Geometry check sheet. Reference: the model listing, model coordinates, mm. A direction names the side the tool comes from. Give positions to 0.01 mm unless a question says otherwise; leave off trailing zeros. Loops run counter-clockwise (first coordinate to the right, second up) from the corner with the lowest first, then second, coordinate; pieces in that order, holes last. Notation, with made-up numbers: (17.5, -1) - (62.5, -1) arc R10 cw to (62.5, 10) - close; hole circle Ø9 at (-14, 57). An arc over 180 degrees is marked (long way). One line per question, with ' | ' between items. Start each with the question number.
from build123d import *

# Parameters (mm, degrees)
SKETCH1_R           = 7.5
SKETCH1_W           = 30
SKETCH1_H           = 3
SKETCH1_W_2         = 3
SKETCH1_H_2         = 30
BOSS_EXTRUDE2_DEPTH = 70


with BuildPart() as part:
    # Sketch1 → Boss-Extrude2 (new body)
    with BuildSketch(Plane.XY):
        Circle(SKETCH1_R)
        Rectangle(SKETCH1_W, SKETCH1_H)
        Rectangle(SKETCH1_W_2, SKETCH1_H_2)
    extrude(amount=BOSS_EXTRUDE2_DEPTH)


solid = part.part
(1) Material ranges on line 1 (X direction, y = -12, z = 41); line 2 (X direction, y = 4, z = 6.5), recorded low to high.
(2) Section check B-B, the plane y = -10.5. Record the boundary of the cut face in (x, z), and give its area (3 significant figures).
(3) Section check C-C, the plane x = -6. Record the boundary of the cut face in (y, z), and give its area (3 significant figures).
(4) Tool access check on faces 1 (the face through (-1.5, -11, 35)), 2 (the face through (11, 1.5, 35)), 3 (the face through (1.5, -11, 35)), 4 (the face through (-1.5, 11, 35)). Record the directions out of +Z, -Z, +X, -X, +Y, -Y that give a thin tool (end or side, any length) a straight path to the whole face; none if there is none.
(5) Section check A-A, the plane z = 60. Record the boundary of the cut face in (x, y).
(6) Depth check by flat-ended pin: pin 1 Ø12 at (x, z) = (11.5, 61) entering from -Y; pin 2 Ø12 at (y, z) = (-7, 21) entering from +X; pin 3 Ø4 at (x, z) = (12.5, 27.5) entering from +Y; pin 4 Ø8.5 at (x, z) = (-10.5, 43) entering from +Y. Enter the tip coordinate at first touch or a pass-through.
Numbers:
1) line 1: -1.5 to 1.5 | line 2: -6.34 to 6.34
2) outline: (-1.5, 0) - (1.5, 0) - (1.5, 70) - (-1.5, 70) - close | area: 210 mm^2
3) outline: (-4.5, 0) - (4.5, 0) - (4.5, 70) - (-4.5, 70) - close | area: 630 mm^2
4) face 1: +Z, -Z, -X, -Y | face 2: +Z, -Z, +X, +Y | face 3: +Z, -Z, +X, -Y | face 4: +Z, -Z, -X, +Y
5) outline: (-15, -1.5) - (-7.35, -1.5) arc R7.5 ccw to (-1.5, -7.35) - (-1.5, -15) - (1.5, -15) - (1.5, -7.35) arc R7.5 ccw to (7.35, -1.5) - (15, -1.5) - (15, 1.5) - (7.35, 1.5) arc R7.5 ccw to (1.5, 7.35) - (1.5, 15) - (-1.5, 15) - (-1.5, 7.35) arc R7.5 ccw to (-7.35, 1.5) - (-15, 1.5) - close
6) pin 1: y = -5.1 | pin 2: x = 15 | pin 3: y = 1.5 | pin 4: y = 4.15
